Verification items for the finished model (mm, model axes). Face numbers are marked on the shaded views. A direction names the side the tool comes from. Give positions to 0.01 mm unless a question says otherwise; leave off trailing zeros. Write each loop counter-clockwise with the first axis right and the second up, starting at its lowest first coordinate (ties: lowest second). Pieces come first, ordered by that corner, then holes. Notation, with made-up numbers: (-29.75, -26.5) -> (2.25, -26.5) arc R16 ccw to (2.25, -8.5) -> close; hole circle Ø11 at (-19, -8.5). An arc over 180 degrees is marked (long way). Answer as CSV lines item,"result". Start each with the question number.
1) Tool access check on the marked faces 1, 2, 3 and 4. Record the directions out of +Z, -Z, +X, -X, +Y, -Y that give a thin tool (end or side, any length) a straight path to the whole face; none if there is none.
2) Sectioned sample at C-C on y = 4. Record the cut outline in (x, z), and give its area (3 significant figures).
3) Sectioned sample at D-D on x = 0. Record the cut outline in (y, z).
4) Sectioned sample at B-B on z = 18. Record the cut outline in (x, y), and give its area (3 significant figures).
5) Gauge pin test, flat ends, axial feed: pin 1 Ø1.8 at (x, y) = (-17.5, -18) entering from -Z; pin 2 Ø2.5 at (x, z) = (15.5, -13.5) entering from -Y; pin 3 Ø1.5 at (y, z) = (7, -36) entering from -X. Record the tip position at first contact, or that the pin passes through.
6) Mould release check, pull along Z, two halves, no side actions. Record for the marked faces 5, 6 and 7: released by +Z, released by -Z, zero draft, split by the parting line, or undercut.
7) Sectioned sample at A-A on y = -2. Record the cut outline in (x, z).
8) Material ranges on L1, parallel to X at y = 15, z = -15; L2, parallel to Z at x = 14, y = -8.5; L3, parallel to Y at x = -7.5, z = -25, recorded low to high.
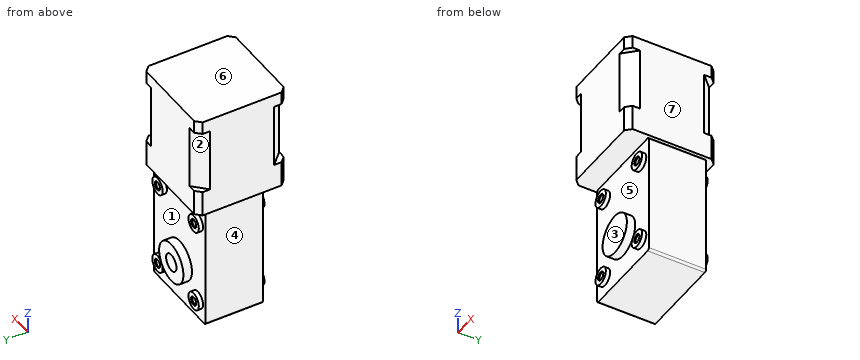
```python
from build123d import *

# Parameters (mm, degrees)
SKETCH_1_W                  = 42
SKETCH_1_H                  = 42
EXTRUDE_1_DEPTH             = 42
CUT_EXTRUDE_1_DEPTH         = 30
CHAMFER_2_SIZE              = 2.5
EXTRUDE_2_DEPTH             = 6
SKETCH_4_W                  = 40
SKETCH_4_H                  = 26.8
EXTRUDE_3_DEPTH             = 58
CUT_EXTRUDE_2_DEPTH         = 58
SKETCH_6_R                  = 9.4
EXTRUDE_4_DEPTH             = 4
SKETCH_7_R                  = 4
EXTRUDE_5_DEPTH             = 2
SKETCH_8_R                  = 4
CUT_EXTRUDE_3_DEPTH         = 14
HOLE_WIZARD_M4_1_AT_2_COUNT = 2
HOLE_WIZARD_M4_1_AT_2_PITCH = 28
HOLE_WIZARD_M4_1_AT_3_COUNT = 2
HOLE_WIZARD_M4_1_AT_3_PITCH = 48.826222463
HOLE_WIZARD_M4_1_AT_4_COUNT = 2
HOLE_WIZARD_M4_1_AT_4_PITCH = 40
SKETCH_11_R                 = 9.4
CUT_EXTRUDE_4_DEPTH         = 0.1


with BuildPart() as part:
    # 스케치1 → 보스-돌출1 (new body)
    with BuildSketch(Plane.XY):
        Rectangle(SKETCH_1_W, SKETCH_1_H)
    extrude(amount=EXTRUDE_1_DEPTH)

    # 스케치2 → 컷-돌출1 (cut)
    with BuildSketch(Plane.XY.offset(36)):
        Polygon((-21, -21), (-15, -21), (-21, -15), align=None)
        Polygon((-21, 21), (-21, 15), (-15, 21), align=None)
        Polygon((21, 21), (15, 21), (21, 15), align=None)
        Polygon((21, -21), (21, -15), (15, -21), align=None)
    extrude(amount=-CUT_EXTRUDE_1_DEPTH, mode=Mode.SUBTRACT)

    # 모따기2
    chamfer_2_edges = [part.edges().sort_by_distance(p)[0] for p in [
        (21, -21, 3),
        (-21, -21, 3),
        (21, 21, 3),
        (-21, 21, 3),
        (21, -21, 39),
        (-21, -21, 39),
        (-21, 21, 39),
        (21, 21, 39),
    ]]
    chamfer(chamfer_2_edges, length=CHAMFER_2_SIZE)

    # 스케치3 → 보스-돌출2 (add)
    with BuildSketch(Plane(origin=(0, 0, 0), x_dir=(-1, 0, 0), z_dir=(0, 0, -1))):
        Polygon((-18.5, 21), (-21, 18.5), (-21, -18.5), (-18.5, -21), (18.5, -21), (21, -18.5), (21, 18.5), (18.5, 21), align=None)
    extrude(amount=EXTRUDE_2_DEPTH)

    # 스케치4 → 보스-돌출3 (add)
    with BuildSketch(Plane(origin=(0, 0, -6), x_dir=(-1, 0, 0), z_dir=(0, 0, -1))):
        with Locations((0, 3.1)):
            Rectangle(SKETCH_4_W, SKETCH_4_H)
    extrude(amount=EXTRUDE_3_DEPTH)

    # 스케치5 → 컷-돌출2 (cut)
    with BuildSketch(Plane(origin=(0, 16.5, 0), x_dir=(1, 0, 0), z_dir=(0, 1, 0))):
        with BuildLine():
            ThreePointArc((-20, 63), (-19.707106781, 63.707106781), (-19, 64))
            Line((-19, 64), (-20, 64))
            Line((-20, 64), (-20, 63))
        make_face()
        with BuildLine():
            Line((20, 64), (19, 64))
            ThreePointArc((19, 64), (19.707106781, 63.707106781), (20, 63))
            Line((20, 63), (20, 64))
        make_face()
        with BuildLine():
            ThreePointArc((-19, 6), (-19.707106781, 6.292893219), (-20, 7))
            Line((-20, 7), (-20, 6))
            Line((-20, 6), (-19, 6))
        make_face()
        with BuildLine():
            Line((20, 6), (20, 7))
            ThreePointArc((20, 7), (19.707106781, 6.292893219), (19, 6))
            Line((19, 6), (20, 6))
        make_face()
    extrude(amount=-CUT_EXTRUDE_2_DEPTH, mode=Mode.SUBTRACT)

    # 스케치6 → 보스-돌출4 (add)
    with BuildSketch(Plane(origin=(0, 16.5, 0), x_dir=(1, 0, 0), z_dir=(0, 1, 0))):
        with Locations((0, 44)):
            Circle(SKETCH_6_R)
    extrude_4 = extrude(amount=EXTRUDE_4_DEPTH)

    # 스케치7 → 보스-돌출5 (add)
    with BuildSketch(Plane(origin=(0, 16.5, 0), x_dir=(1, 0, 0), z_dir=(0, 1, 0))):
        with Locations((14, 55)):
            Circle(SKETCH_7_R)
        with Locations((-14, 55)):
            Circle(SKETCH_7_R)
        with Locations((-14, 15)):
            Circle(SKETCH_7_R)
        with Locations((14, 15)):
            Circle(SKETCH_7_R)
    extrude_5 = extrude(amount=EXTRUDE_5_DEPTH)

    # 스케치8 → 컷-돌출3 (cut)
    with BuildSketch(Plane(origin=(0, 20.5, 0), x_dir=(1, 0, 0), z_dir=(0, 1, 0))):
        with Locations(Location((0, 44, 0), (0, 0, 180))):
            Circle(SKETCH_8_R)
    extrude(amount=-CUT_EXTRUDE_3_DEPTH, mode=Mode.SUBTRACT)

    # 스케치10 → M4 나사 구멍1 (revolve, cut)
    with BuildSketch(Plane(origin=(-14, 18.5, -55), x_dir=(0, 0, 1), z_dir=(1, 0, 0))):
        Polygon((0, 0), (0, 12.491420021), (1.65, 11.5), (1.65, 0.375), (2.025, 0), align=None)
    hole_wizard_m4_1 = revolve(axis=Axis((-14, 24.85, -55), (0, -1, 0)), mode=Mode.SUBTRACT)

    # M4 나사 구멍1 at 2: M4 나사 구멍1 ×2
    with Locations(*[(i * HOLE_WIZARD_M4_1_AT_2_PITCH, 0, 0) for i in range(1, HOLE_WIZARD_M4_1_AT_2_COUNT)]):
        add(hole_wizard_m4_1, mode=Mode.SUBTRACT)

    # M4 나사 구멍1 at 3: M4 나사 구멍1 ×2
    with Locations(*[Vector(0.5734623443633283, 0, 0.8192319205190405) * (i * HOLE_WIZARD_M4_1_AT_3_PITCH) for i in range(1, HOLE_WIZARD_M4_1_AT_3_COUNT)]):
        add(hole_wizard_m4_1, mode=Mode.SUBTRACT)

    # M4 나사 구멍1 at 4: M4 나사 구멍1 ×2
    with Locations(*[(0, 0, i * HOLE_WIZARD_M4_1_AT_4_PITCH) for i in range(1, HOLE_WIZARD_M4_1_AT_4_COUNT)]):
        add(hole_wizard_m4_1, mode=Mode.SUBTRACT)

    # 대칭 복사1: 보스-돌출4, 보스-돌출5, M4 나사 구멍1 across plane
    add(extrude_4.mirror(Plane.ZX.offset(3.1)))
    add(extrude_5.mirror(Plane.ZX.offset(3.1)))
    add(hole_wizard_m4_1.mirror(Plane.ZX.offset(3.1)), mode=Mode.SUBTRACT)

    # 대칭 복사1 copy 1 sketch → 대칭 복사1 copy 1 (revolve, cut)
    with BuildSketch(Plane(origin=(14, -12.3, -55), x_dir=(0, 0, 1), z_dir=(1, 0, 0))):
        Polygon((0, 0), (0, -12.491420021), (1.65, -11.5), (1.65, -0.375), (2.025, 0), align=None)
    revolve(axis=Axis((14, -18.65, -55), (0, -1, 0)), mode=Mode.SUBTRACT)

    # 대칭 복사1 copy 2 sketch → 대칭 복사1 copy 2 (revolve, cut)
    with BuildSketch(Plane(origin=(14, -12.3, -15), x_dir=(0, 0, 1), z_dir=(1, 0, 0))):
        Polygon((0, 0), (0, -12.491420021), (1.65, -11.5), (1.65, -0.375), (2.025, 0), align=None)
    revolve(axis=Axis((14, -18.65, -15), (0, -1, 0)), mode=Mode.SUBTRACT)

    # 대칭 복사1 copy 3 sketch → 대칭 복사1 copy 3 (revolve, cut)
    with BuildSketch(Plane(origin=(-14, -12.3, -15), x_dir=(0, 0, 1), z_dir=(1, 0, 0))):
        Polygon((0, 0), (0, -12.491420021), (1.65, -11.5), (1.65, -0.375), (2.025, 0), align=None)
    revolve(axis=Axis((-14, -18.65, -15), (0, -1, 0)), mode=Mode.SUBTRACT)

    # 스케치11 → 컷-돌출4 (cut)
    with BuildSketch(Plane.XZ.offset(14.3)):
        with Locations(Location((0, -44, 0), (0, 0, 180))):
            Circle(SKETCH_11_R)
    extrude(amount=-CUT_EXTRUDE_4_DEPTH, mode=Mode.SUBTRACT)


solid = part.part
```
Ans:
1,face 1,"+Y"
1,face 2,"-X, +Y"
1,face 3,"-Z, +X, -X, -Y"
1,face 4,"-Z, -X, +Y, -Y"
2,outline,"(-21, -6) -> (-19, -6) arc R1 ccw to (-20, -7) -> (-20, -63) arc R1 ccw to (-19, -64) -> (19, -64) arc R1 ccw to (20, -63) -> (20, -7) arc R1 ccw to (19, -6) -> (21, -6) -> (21, 42) -> (-21, 42) -> close"
2,area,"4,340 mm²"
3,outline,"(-21, -6) -> (-10.3, -6) -> (-10.3, -34.6) -> (-14.2, -34.6) -> (-14.2, -53.4) -> (-10.3, -53.4) -> (-10.3, -64) -> (16.5, -64) -> (16.5, -53.4) -> (20.5, -53.4) -> (20.5, -48) -> (6.5, -48) -> (6.5, -40) -> (20.5, -40) -> (20.5, -34.6) -> (16.5, -34.6) -> (16.5, -6) -> (21, -6) -> (21, 42) -> (-21, 42) -> close"
4,outline,"(-21, -15) -> (-15, -21) -> (15, -21) -> (21, -15) -> (21, 15) -> (15, 21) -> (-15, 21) -> (-21, 15) -> close"
4,area,"1,690 mm²"
5,pin 1,"stops at z = -6"
5,pin 2,"stops at y = -12.3"
5,pin 3,"stops at x = -20"
6,face 5,"undercut"
6,face 6,"released by +Z"
6,face 7,"zero draft"
7,outline,"(-21, -6) -> (-19, -6) arc R1 ccw to (-20, -7) -> (-20, -63) arc R1 ccw to (-19, -64) -> (19, -64) arc R1 ccw to (20, -63) -> (20, -7) arc R1 ccw to (19, -6) -> (21, -6) -> (21, 42) -> (-21, 42) -> close; hole circle Ø3.3 at (-14, -55); hole circle Ø3.3 at (-14, -15); hole circle Ø3.3 at (14, -55); hole circle Ø3.3 at (14, -15)"
8,L1,"x = -20 to -15.65, -12.35 to 12.35, 15.65 to 20"
8,L2,"z = -64 to -56.65, -53.35 to -16.65, -13.35 to 42"
8,L3,"y = -10.3 to 16.5"
